Source: CAD feature listing. Evaluate the final solid. Frame: model axes, mm. Face numbers are marked on the shaded views. A direction names the side the tool comes from. Coordinates: 2 decimals unless noted, no trailing zeros. Order: outer loops, then holes, each group sorted by start corner. A loop starts at its lowest first (then second) coordinate and runs counter-clockwise, first axis right, second up.
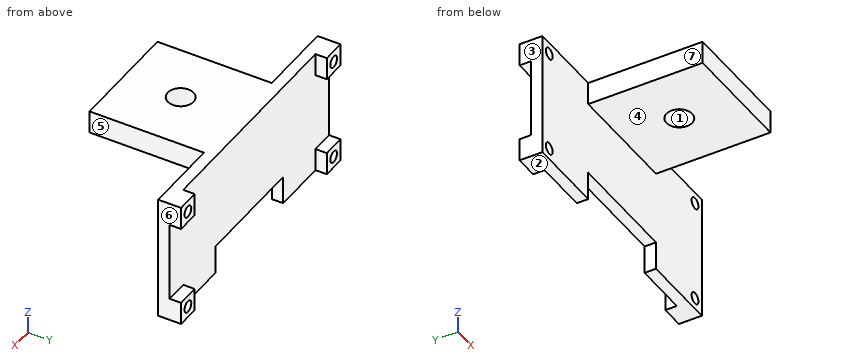
Autodesk Fusion 360 part; units mm, degrees
sketch "Sketch1" plane through (0, 0, 0) normal (0, 1, 0) x (1, 0, 0)
  line L0 (-21.5, 9) -> (21.5, 9) construction
  line L1 (21.5, 9) -> (21.5, -9) construction
  line L2 (21.5, -9) -> (-21.5, -9) construction
  line L3 (-21.5, -9) -> (-21.5, 9) construction
  line L4 (-21.5, 9) -> (21.5, -9) construction
  circle A0 centre (-21.5, -9) radius 1
  circle A1 centre (21.5, -9) radius 1
  circle A2 centre (-21.5, 9) radius 1
  circle A3 centre (21.5, 9) radius 1
  line L5 (23.5, -11) -> (-23.5, -11)
  line L6 (-23.5, -11) -> (-23.5, 11)
  line L7 (-23.5, 11) -> (23.5, 11)
  line L8 (23.5, 11) -> (23.5, -11)
  line L9 (-23.5, 11) -> (-19.5, 11)
  line L10 (-19.5, 11) -> (-19.5, 7)
  line L11 (-19.5, 7) -> (-23.5, 7)
  line L12 (-23.5, 7) -> (-23.5, 11)
  line L13 (-23.5, -11) -> (-19.5, -11)
  line L14 (-19.5, -11) -> (-19.5, -7)
  line L15 (-19.5, -7) -> (-23.5, -7)
  line L16 (-23.5, -7) -> (-23.5, -11)
  line L17 (23.5, 11) -> (19.5, 11)
  line L18 (19.5, 11) -> (19.5, 7)
  line L19 (19.5, 7) -> (23.5, 7)
  line L20 (23.5, 7) -> (23.5, 11)
  line L21 (23.5, -11) -> (19.5, -11)
  line L22 (19.5, -11) -> (19.5, -7)
  line L23 (19.5, -7) -> (23.5, -7)
  line L24 (23.5, -7) -> (23.5, -11)
  line L25 (-10, 11) -> (10, 11)
  line L26 (10, 11) -> (10, 6)
  line L27 (10, 6) -> (-10, 6)
  line L28 (-10, 6) -> (-10, 11)
  dimension "d1" = 43
  dimension "d2" = 18
  dimension "d3" = 2
  dimension "d4" = 2
  dimension "d5" = 2
  dimension "d6" = 2
  dimension "d7" = -2
  dimension "d8" = 4
  dimension "d9" = 4
  dimension "d10" = 4
  dimension "d11" = 4
  dimension "d12" = 4
  dimension "d13" = 4
  dimension "d14" = 4
  dimension "d15" = 4
  dimension "d28" = 20
  dimension "d29" = 5
extrude "Extrude1" add sketch "Sketch1" against normal blind 2 contours L5 L8 L21 L22 L23 L24 | L5 L6 L7 L8 L10 L11 L14 L15 L18 L19 L22 L23 L26 L27 L28 | L5 L6 L13 L14 L15 L16 | L7 L8 L17 L18 L19 L20 | L6 L7 L9 L10 L11 L12
extrude "Extrude2" add sketch "Sketch1" along normal blind 2 contours L5 L8 L21 L22 L23 L24 | L5 L6 L13 L14 L15 L16 | L7 L8 L17 L18 L19 L20 | L6 L7 L9 L10 L11 L12
sketch "Sketch2" plane through (0, -2, 0) normal (0, -1, 0) x (1, 0, 0)
  circle A0 centre (-21.5, 9) radius 1
  circle A1 centre (-21.5, -9) radius 1
  circle A2 centre (21.5, 9) radius 1
  circle A3 centre (21.5, -9) radius 1
  line L0 (23.5, -11) -> (23.5, 11)
  line L1 (23.5, 11) -> (-23.5, 11)
  line L2 (-23.5, 11) -> (-23.5, -11)
  line L3 (10, -11) -> (23.5, -11)
  line L4 (-10, 11) -> (10, 11)
  line L5 (10, 11) -> (10, -9)
  line L6 (10, -9) -> (-10, -9)
  line L7 (-10, -9) -> (-10, 11)
  line L8 (23.5, 11) -> (-23.5, 11)
  line L9 (-10, 11) -> (10, 11)
  line L10 (10, 11) -> (10, 7)
  line L11 (10, 7) -> (-10, 7)
  line L12 (-10, 7) -> (-10, 11)
  line L13 (10, -6) -> (10, -11)
  line L14 (-23.5, -11) -> (-10, -11)
  line L15 (-10, -11) -> (-10, -6)
  line L16 (-10, -6) -> (10, -6)
  dimension "d20" = 20
  dimension "d21" = 20
  dimension "d22" = 4
extrude "Extrude3" add sketch "Sketch2" along normal blind 20 contours L1 L4 L5 L7 L8 L9 L10 L11 L12
sketch "Sketch3" plane through (0, 0, 7) normal (0, 0, -1) x (-1, 0, 0)
  line L0 (10, -2) -> (-10, -2)
  line L1 (-10, -2) -> (-10, -22)
  line L2 (-10, -22) -> (10, -22)
  line L3 (10, -22) -> (10, -2)
  circle A0 centre (0, -12) radius 2.25
  line L4 (10, -22) -> (-10, -2) construction
  dimension "d25" = 4.5
extrude "Extrude4" cut sketch "Sketch3" against normal blind 4 contours A0
1. Ray query, line 1 (X direction, y = 1.2, z = 9); line 2 (X direction, y = -0.5, z = 9); line 3 (Z direction, x = 21.5, y = -1.2). Return the intervals inside material, ascending.
Findings:
line 1: x = -23.5 to -22.5, -20.5 to -19.5, 19.5 to 20.5, 22.5 to 23.5
line 2: x = -23.5 to -22.5, -20.5 to 20.5, 22.5 to 23.5
line 3: z = -11 to -10, -8 to 8, 10 to 11
2. Section query A-A on y = -12. Return loops of the section in (x, z), plus the area to 3 significant figures.
Findings:
outline: (-10, 7) - (-2.25, 7) - (-2.25, 11) - (-10, 11) - close; (2.25, 7) - (10, 7) - (10, 11) - (2.25, 11) - close
area: 62.0 mm2
3. Section query D-D on x = -21.5. Return loops of the section in (y, z).
Findings:
outline: (-2, -11) - (2, -11) - (2, -10) - (-2, -10) - close; (-2, -8) - (2, -8) - (2, -7) - (0, -7) - (0, 7) - (2, 7) - (2, 8) - (-2, 8) - close; (-2, 10) - (2, 10) - (2, 11) - (-2, 11) - close
4. Pin query (flat end, axial travel): P1, Ø10, axis at x = -3, y = -9.5, coming from the -Z side; P2, Ø3, axis at x = 21.5, z = 9, coming from the -Y side; P3, Ø4, axis at x = 17.5, z = -6.5, coming from the +Y side. Return the tip coordinate at first contact, or that it passes through.
Findings:
P1: stops at z = 7
P2: stops at y = -2
P3: stops at y = 0
5. Draft query along Y for the marked faces 1 and 2. Return one class per face: released by +Y, released by -Y, zero draft, split by the parting line, or undercut.
Findings:
face 1: undercut
face 2: zero draft
6. Section query B-B on x = 1.5. Return loops of the section in (y, z), plus the area to 3 significant figures.
Findings:
outline: (-22, 7) - (-13.68, 7) - (-13.68, 11) - (-22, 11) - close; (-10.32, 7) - (-2, 7) - (-2, -6) - (0, -6) - (0, 11) - (-10.32, 11) - close
area: 101 mm2
7. Section query C-C on z = -6.5. Return loops of the section in (x, y).
Findings:
outline: (-23.5, -2) - (-10, -2) - (-10, 0) - (-23.5, 0) - close; (10, -2) - (23.5, -2) - (23.5, 0) - (10, 0) - close
8. Access query for the marked faces 3, 4, 5, 6 and 7. Directions: +Z, -Z, +X, -X, +Y, -Y. A direction counts if a zero-diameter tool reaches every point of the face in a straight line with its end or side. Return the directions, or none.
Findings:
face 3: +Z, -Z, -X, +Y, -Y
face 4: -Z, +X, -X, -Y
face 5: +Z, -Z, +X, -Y
face 6: +Z, -Z, +X, +Y, -Y
face 7: +Z, -Z, -X, -Y
